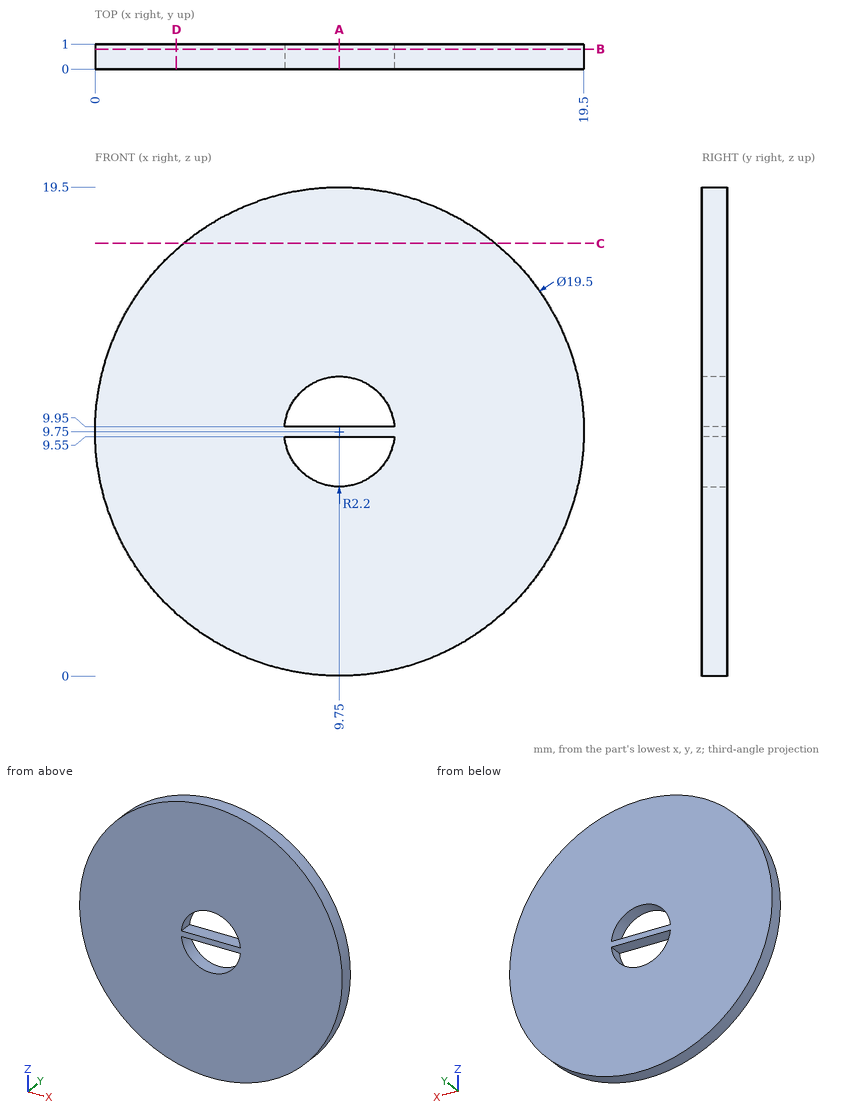
The drawing under review shows one solid part. Ordinate dimensions are in mm from its lowest x, y, z. Round coordinates to 2 decimals unless told otherwise and drop trailing zeros. Loops run counter-clockwise (first coordinate to the right, second up) from the corner with the lowest first, then second, coordinate; pieces in that order, holes last. Notation, with made-up numbers: (-4, 71.25) - (37, 71.25) arc R14 cw to (37, 79.25) - close; hole circle Ø2 at (33.25, 9.25). An arc over 180 degrees is marked (long way). Use a Markdown table: item, result. Add a question column.
Q1. For probe 1 along Z at (x, y) = (8.75, 0.25); probe 2 along Z at (x, y) = (10.5, 0.3); probe 3 along X at (y, z) = (0.1, 10.25), list the stretches that pass through material, from the lowest coordinate up.
Q2. Add section A-A (x = 9.75). State the section outline as (y, z) points, plus the area to 3 significant figures.
Q3. Add section C-C (z = 17.25). State the section outline as (x, y) points.
Q4. Add section B-B (y = 0.8). State the section outline as (x, z) points.
Q5. Add section D-D (x = 3.25). State the section outline as (y, z) points.
Worked answers:
| question | item | result |
|---|---|---|
| 1 | probe 1 | 0.05 to 7.79, 9.55 to 9.95, 11.71 to 19.45 |
| 1 | probe 2 | 0.03 to 7.68, 9.55 to 9.95, 11.82 to 19.47 |
| 1 | probe 3 | 0.01 to 7.61, 11.89 to 19.49 |
| 2 | outline | (0, 0) - (1, 0) - (1, 7.55) - (0, 7.55) - close; (0, 9.55) - (1, 9.55) - (1, 9.95) - (0, 9.95) - close; (0, 11.95) - (1, 11.95) - (1, 19.5) - (0, 19.5) - close |
| 2 | area | 15.5 mm² |
| 3 | outline | (3.52, 0) - (15.98, 0) - (15.98, 1) - (3.52, 1) - close |
| 4 | outline | circle Ø19.5 at (9.75, 9.75); hole (7.56, 9.55) arc R2.2 ccw to (11.94, 9.55) - close; hole (7.56, 9.95) - (11.94, 9.95) arc R2.2 ccw to start |
| 5 | outline | (0, 2.48) - (1, 2.48) - (1, 17.02) - (0, 17.02) - close |
